Read the model definition and answer for the solid it produces. Units are mm, in the model's axes. Face numbers are marked on the shaded views. A direction names the side the tool comes from. Coordinates: 2 decimals unless noted, no trailing zeros. Write each loop counter-clockwise with the first axis right and the second up, starting at its lowest first coordinate (ties: lowest second). Pieces come first, ordered by that corner, then holes.
(1) Given pin 1 (1.5 mm diameter, centred on x = -21.5, y = -66, fed in from +Z), flat-ended and moving along its own axis, determine where the tip first touches the part or whether it passes through.
(2) Section B-B on y = -48.5 is taken. Write down the section's boundary in (x, z), then the cut area to 3 significant figures.
(3) Find the intervals of material crossed by probe 1 along X at (y, z) = (63, 25.5); probe 2 along Y at (x, z) = (2, 62.5); probe 3 along Z at (x, y) = (-48.5, 44.5), in increasing order.
(4) Section A-A on z = 22 is taken. Write down the section's boundary in (x, y), then the cut area to 3 significant figures.
(5) Section C-C on x = 53.5 is taken. Write down the section's boundary in (y, z), then the cut area to 3 significant figures.
(6) Section D-D on y = 2.5 is taken. Write down the section's boundary in (x, z), then the cut area to 3 significant figures.
(7) Which of the six approach directions +Z, -Z, +X, -X, +Y, -Y give full straight-line access (tool end or side, diameter ignored) to the marked faces 1 and 2?
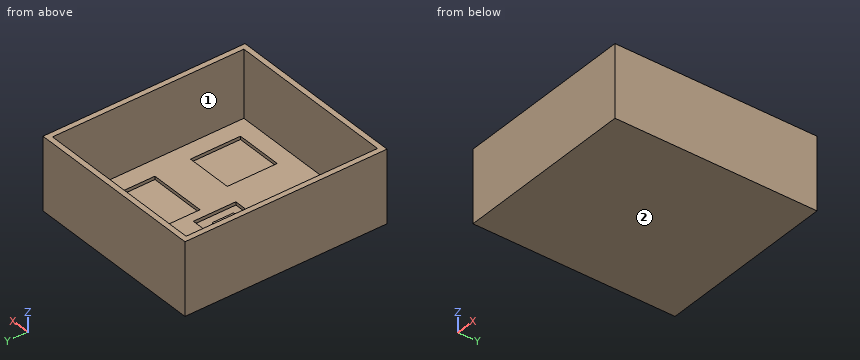
Autodesk Inventor part; units mm, degrees
ref_plane "YZ Plane" through (0, 0, 0) normal (1, 0, 0) x (0, 1, 0)
ref_plane "XZ Plane" through (0, 0, 0) normal (0, 1, 0) x (-1, 0, 0)
ref_plane "XY Plane" through (0, 0, 0) normal (0, 0, 1) x (1, 0, 0)
sketch "Sketch1" plane through (0, 0, 0) normal (0, 0, 1) x (1, 0, 0)
  line L0 (90, -90) -> (-70, -90)
  line L1 (-70, -90) -> (-70, 90)
  line L2 (-70, 90) -> (90, 90)
  line L3 (90, 90) -> (90, -90)
  line L4 (95, 95) -> (-75, 95)
  line L5 (-75, 95) -> (-75, -95)
  line L6 (-75, -95) -> (95, -95)
  line L7 (95, -95) -> (95, 95)
  point P0 (0, 0)
  dimension "d45" = 180
  dimension "d46" = 5
  dimension "d61" = 70
  dimension "d62" = 90
  dimension "d63" = 5
extrude "Extrusion1" add sketch "Sketch1" along normal blind 68
extrude "Extrusion2" add sketch "Sketch1" along normal blind 5 contours L0 L1 L2 L3
sketch "Sketch2" plane through (0, 0, 5) normal (0, 0, 1) x (1, 0, 0)
  line L0 (29.7141, -27.0003) -> (73.7141, -27.0003)
  line L1 (73.7141, -27.0003) -> (73.7141, -74.0003)
  line L2 (73.7141, -74.0003) -> (29.7141, -74.0003)
  line L3 (29.7141, -74.0003) -> (29.7141, -27.0003)
  circle A0 centre (0, 0) radius 150 construction
  line L4 (72.9434, 76.0673) -> (72.9434, 7.0673)
  line L5 (72.9434, 7.0673) -> (18.9434, 7.0673)
  line L6 (18.9434, 7.0673) -> (18.9434, 76.0673)
  line L7 (18.9434, 76.0673) -> (72.9434, 76.0673)
  line L8 (45.9434, 76.0673) -> (45.9434, 7.0673) construction
  line L9 (-70, -90) -> (90, -90)
  line L10 (90, -90) -> (90, 90)
  line L11 (90, 90) -> (-70, 90)
  line L12 (-70, 90) -> (-70, -90)
  line L13 (90, 90) -> (90, -90)
  line L14 (-25.5, -10) -> (0.5, -10)
  line L15 (0.5, -10) -> (0.5, 10)
  line L16 (0.5, 10) -> (-25.5, 10)
  line L17 (-25.5, 10) -> (-25.5, -10)
  line L18 (-35.5, -20) -> (10.5, -20)
  line L19 (10.5, -20) -> (10.5, 20)
  line L20 (10.5, 20) -> (-35.5, 20)
  line L21 (-35.5, 20) -> (-35.5, -20)
  point P0 (51.7141, -50.5003)
  point P1 (73.7141, -50.5003)
  point P2 (51.7141, -27.0003)
  point P3 (45.9434, 41.5673)
  dimension "d6" = 47
  dimension "d7" = 44
  dimension "d8" = 54
  dimension "d9" = 69
  dimension "d47" = 160
  dimension "d48" = 160
  dimension "d54" = 26
  dimension "d55" = 20
  dimension "d56" = 46
  dimension "d57" = 40
  dimension "d58" = 0.5
  dimension "d59" = 10
  dimension "d60" = 10
extrude "Extrusion3" cut sketch "Sketch2" against normal blind 1.5 contours L0 L1 L2 L3 | L4 L5 L6 L7
extrude "Extrusion4" cut sketch "Sketch2" against normal blind 3 contours L0 L1 L2 L3 | L4 L5 L6 L7 | L21 L20 L19 L18
properties part number "Shooting Mechanism Box" material "Glass"
Response:
1. pin 1: stops at z = 5
2. outline: (-75, 0) - (95, 0) - (95, 68) - (90, 68) - (90, 5) - (73.71, 5) - (73.71, 2) - (29.71, 2) - (29.71, 5) - (-70, 5) - (-70, 68) - (-75, 68) - close
2. area: 1,350 mm2
3. probe 1: x = -75 to -70, 90 to 95
3. probe 2: y = -95 to -90, 90 to 95
3. probe 3: z = 0 to 5
4. outline: (-75, -95) - (95, -95) - (95, 95) - (-75, 95) - close; hole (-70, -90) - (90, -90) - (90, 90) - (-70, 90) - close
4. area: 3,500 mm2
5. outline: (-95, 0) - (95, 0) - (95, 68) - (90, 68) - (90, 5) - (76.07, 5) - (76.07, 2) - (7.07, 2) - (7.07, 5) - (-27, 5) - (-27, 2) - (-74, 2) - (-74, 5) - (-90, 5) - (-90, 68) - (-95, 68) - close
5. area: 1,230 mm2
6. outline: (-75, 0) - (95, 0) - (95, 68) - (90, 68) - (90, 5) - (10.5, 5) - (10.5, 2) - (0.5, 2) - (0.5, 5) - (-25.5, 5) - (-25.5, 2) - (-35.5, 2) - (-35.5, 5) - (-70, 5) - (-70, 68) - (-75, 68) - close
6. area: 1,420 mm2
7. face 1: +Z
7. face 2: -Z, +X, -X, +Y, -Y
